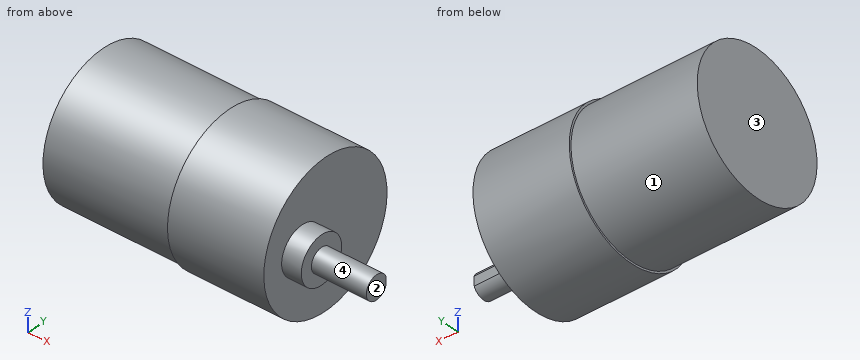
from build123d import *

# Parameters (mm, degrees)
SKETCH2_R           = 6.0000007
BOSS_EXTRUDE1_DEPTH = 4.99999
BOSS_EXTRUDE2_DEPTH = 13.9999974


with BuildPart() as part:
    # Sketch1 → Revolve1 (revolve)
    with BuildSketch(Plane.XY, mode=Mode.PRIVATE) as revolve1_sk:
        Polygon((28.321, 0), (28.321, 18.288), (3.80803947, 18.288), (3.80803947, 17.78), (-28.321, 17.78), (-28.321, 0), align=None)
    revolve(revolve1_sk.sketch.rotate(Axis((-37.449530368, 0, 0), (1, 0, 0)), 90), axis=Axis((-37.449530368, 0, 0), (1, 0, 0)))

    # Sketch2 → Boss-Extrude1 (add)
    with BuildSketch(Plane(origin=(28.321, 0, 0), x_dir=(0, 0, -1), z_dir=(1, 0, 0))):
        with Locations(Location((0, -7.00024, 0), (0, 0, 180))):
            Circle(SKETCH2_R)
    extrude(amount=BOSS_EXTRUDE1_DEPTH)

    # Sketch3 → Boss-Extrude2 (add)
    with BuildSketch(Plane(origin=(33.32099, 0, 0), x_dir=(0, 0, -1), z_dir=(1, 0, 0))):
        with BuildLine():
            Line((-1.198955483, -4.2502455), (1.198955483, -4.2502455))
            ThreePointArc((1.198955483, -4.2502455), (0, -10.000234), (-1.198955483, -4.2502455))
        make_face()
    extrude(amount=BOSS_EXTRUDE2_DEPTH)


solid = part.part
Source: CAD feature listing. Evaluate the final solid. Frame: model axes, mm. Face numbers are marked on the shaded views. A direction names the side the tool comes from. Round coordinates to 2 decimals unless told otherwise and drop trailing zeros. Order: outer loops, then holes, each group sorted by start corner. A loop starts at its lowest first (then second) coordinate and runs counter-clockwise, first axis right, second up. Notation, with made-up numbers: (72.25, 46.5) -> (103.25, 46.5) arc R24 cw to (103.25, 63.5) -> close; hole circle Ø10 at (20, 30). An arc over 180 degrees is marked (long way). Answer as CSV lines item,"result".
Item 1: Section D-D, the plane z = 10. Return loops of the section in (x, y).
A:
outline,"(-28.32, -14.7) -> (3.81, -14.7) -> (3.81, -15.31) -> (28.32, -15.31) -> (28.32, 15.31) -> (3.81, 15.31) -> (3.81, 14.7) -> (-28.32, 14.7) -> close"
Item 2: Section B-B, the plane z = 0. Return loops of the section in (x, y), plus the area to 3 significant figures.
A:
outline,"(-28.32, -17.78) -> (3.81, -17.78) -> (3.81, -18.29) -> (28.32, -18.29) -> (28.32, -13) -> (33.32, -13) -> (33.32, -10) -> (47.32, -10) -> (47.32, -4.25) -> (33.32, -4.25) -> (33.32, -1) -> (28.32, -1) -> (28.32, 18.29) -> (3.81, 18.29) -> (3.81, 17.78) -> (-28.32, 17.78) -> close"
area,"2,180 mm²"
Item 3: Reachability of the marked faces 3 and 4 from +Z, -Z, +X, -X, +Y, -Y: full face, straight path, thin tool, end or side. Return the list, or none.
A:
face 3,"+Z, -Z, -X, +Y, -Y"
face 4,"+X"
Item 4: Section A-A, the plane y = 0. Return loops of the section in (x, z).
A:
outline,"(-28.32, -17.78) -> (3.81, -17.78) -> (3.81, -18.29) -> (28.32, -18.29) -> (28.32, 18.29) -> (3.81, 18.29) -> (3.81, 17.78) -> (-28.32, 17.78) -> close"
Item 5: Pull-direction query (Z, two-part tool) for the marked faces 1 and 2; classes: pulls with the +Z half, pulls with the -Z half, needs draft (parallel to the pull), parting line crosses it, or undercut.
A:
face 1,"parting line crosses it"
face 2,"needs draft"
Item 6: Line query: L1, parallel to X at y = -1.5, z = -8; L2, parallel to X at y = -9, z = -2.5; L3, parallel to Z at x = -5, y = -12. Output: solid intervals per line, ascending.
A:
L1,"-28.32 to 28.32"
L2,"-28.32 to 33.32"
L3,"-13.12 to 13.12"
Item 7: Section C-C, the plane x = 5. Return loops of the section in (y, z), plus the area to 3 significant figures.
A:
outline,"circle Ø36.58 at (0, 0)"
area,"1,050 mm²"
Item 8: Pin query (flat end, axial travel): pin 1 Ø1.9 at (x, z) = (41.5, 0) entering from +Y; pin 2 Ø12 at (x, y) = (27, 6.5) entering from +Z; pin 3 Ø1.5 at (x, y) = (0.5, -9) entering from -Z. Return the tip coordinate at first contact, or that it passes through.
A:
pin 1,"y = -4.25"
pin 2,"z = 18.28"
pin 3,"z = -15.75"
